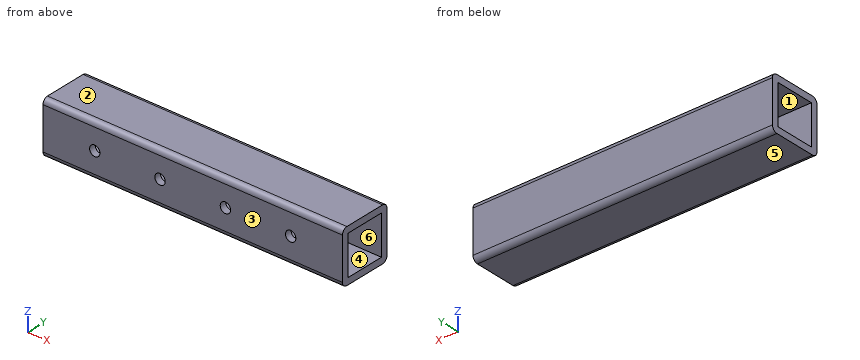
```python
from build123d import *

# Parameters (mm, degrees)
F0_W     = 289.201
F0_H     = 50.8
F1_DEPTH = 50.8
F2_R     = 5
F3_DEPTH = 25.4
F4_W     = 38.1
F4_H     = 38.1
F5_DEPTH = 289.202
F6_R     = 5.08


with BuildPart() as f1:
    # F0 (on Front) → F1 (new body)
    with BuildSketch(Plane.XZ):
        with Locations((-1315.305821, 25.4)):
            Rectangle(F0_W, F0_H)
    extrude(amount=F1_DEPTH)

    # F2 (on face) → F3 (cut)
    with BuildSketch(Plane.XZ.offset(50.8)):
        with Locations((-1346.839321, 25.4)):
            Circle(F2_R)
        with Locations((-1220.705321, 25.4)):
            Circle(F2_R)
        with Locations((-1283.772321, 25.4)):
            Circle(F2_R)
        with Locations((-1409.906321, 25.4)):
            Circle(F2_R)
    extrude(amount=-F3_DEPTH, mode=Mode.SUBTRACT)

    # F4 (on face) → F5 (cut, through all)
    with BuildSketch(Plane(origin=(-1459.906321, 0, 0), x_dir=(0, -1, 0), z_dir=(-1, 0, 0))):
        with Locations((25.4, 25.4)):
            Rectangle(F4_W, F4_H)
    extrude(amount=-F5_DEPTH, mode=Mode.SUBTRACT)

    # F6
    f6_edges = [f1.edges().sort_by_distance(p)[0] for p in [
        (-1315.305821, -50.8, 50.8),
        (-1315.305821, 0, 50.8),
        (-1315.305821, -50.8, 0),
        (-1315.305821, 0, 0),
    ]]
    fillet(f6_edges, radius=F6_R)


solid = f1.part
```
Part model, mm, in its own coordinate system. Face numbers are marked on the shaded views. A direction names the side the tool comes from. Give positions to 0.01 mm unless a question says otherwise; leave off trailing zeros. Write each loop counter-clockwise with the first axis right and the second up, starting at its lowest first coordinate (ties: lowest second). Pieces come first, ordered by that corner, then holes. Notation, with made-up numbers: (43, -11) -> (100, -11) arc R25 cw to (100, 25) -> close; hole circle Ø3 at (33.5, 23.5). An arc over 180 degrees is marked (long way). Put each result on its own line as item: value. Start each with the question number.
Item 1: Pin check, flat tips, straight feed: pin 1 Ø6 at (x, z) = (-1409.91, 25.4) entering from -Y; pin 2 Ø10 at (y, z) = (-39.5, 36) entering from -X. Stop position of each tip, or through.
Item 2: Cut at D-D (z = 25.4). List the corners of the cut face in (x, y).
Item 3: Cut at B-B (y = -10.5). List the corners of the cut face in (x, z).
Item 4: Cut at A-A (z = 42). List the corners of the cut face in (x, y), then the cut area to 3 significant figures.
Item 5: Pull direction Y, two halves, no side cores. Call the marked faces 3, 4, 5 and 6: pulls with the +Y half, pulls with the -Y half, needs draft (parallel to the pull), parting line crosses it, or undercut.
Item 6: Which spindle directions (+Z, -Z, +X, -X, +Y, -Y) get a long thin tool onto all of the face, cutting with end or side? Do the marked faces 1 and 2. Say none if no direction does.
Item 7: Wall check: L1, parallel to X at y = -48, z = 25; L2, parallel to Z at x = -1357.5, y = -43.5; L3, parallel to Y at x = -1203, z = 9.5. Give the ranges that are in metal, low to high. Write a range as [from, to].
Item 8: Cut at C-C (x = -1272). List the corners of the cut face in (y, z), then the cut area to 3 significant figures.
Answer list:
1. pin 1: stops at y = -6.35
1. pin 2: stops at x = -1459.91
2. outline: (-1459.91, -50.8) -> (-1414.91, -50.8) -> (-1414.91, -44.45) -> (-1459.91, -44.45) -> close; (-1459.91, -6.35) -> (-1170.71, -6.35) -> (-1170.71, 0) -> (-1459.91, 0) -> close; (-1404.91, -50.8) -> (-1351.84, -50.8) -> (-1351.84, -44.45) -> (-1404.91, -44.45) -> close; (-1341.84, -50.8) -> (-1288.77, -50.8) -> (-1288.77, -44.45) -> (-1341.84, -44.45) -> close; (-1278.77, -50.8) -> (-1225.71, -50.8) -> (-1225.71, -44.45) -> (-1278.77, -44.45) -> close; (-1215.71, -50.8) -> (-1170.71, -50.8) -> (-1170.71, -44.45) -> (-1215.71, -44.45) -> close
3. outline: (-1459.91, 0) -> (-1170.71, 0) -> (-1170.71, 6.35) -> (-1459.91, 6.35) -> close; (-1459.91, 44.45) -> (-1170.71, 44.45) -> (-1170.71, 50.8) -> (-1459.91, 50.8) -> close
4. outline: (-1459.91, -50.8) -> (-1170.71, -50.8) -> (-1170.71, -44.45) -> (-1459.91, -44.45) -> close; (-1459.91, -6.35) -> (-1170.71, -6.35) -> (-1170.71, 0) -> (-1459.91, 0) -> close
4. area: 3,670 mm2
5. face 3: pulls with the -Y half
5. face 4: undercut
5. face 5: needs draft
5. face 6: undercut
6. face 1: +X, -X
6. face 2: +Z, +X, -X, +Y, -Y
7. L1: x = [-1459.91, -1414.89], [-1404.92, -1351.82], [-1341.86, -1288.76], [-1278.79, -1225.69], [-1215.72, -1170.71]
7. L2: z = [0, 6.35], [44.45, 50.8]
7. L3: y = [-50.8, -44.45], [-6.35, 0]
8. outline: (-50.8, 5.08) arc R5.08 ccw to (-45.72, 0) -> (-5.08, 0) arc R5.08 ccw to (0, 5.08) -> (0, 45.72) arc R5.08 ccw to (-5.08, 50.8) -> (-45.72, 50.8) arc R5.08 ccw to (-50.8, 45.72) -> close; hole (-44.45, 6.35) -> (-6.35, 6.35) -> (-6.35, 44.45) -> (-44.45, 44.45) -> close
8. area: 1,110 mm2
